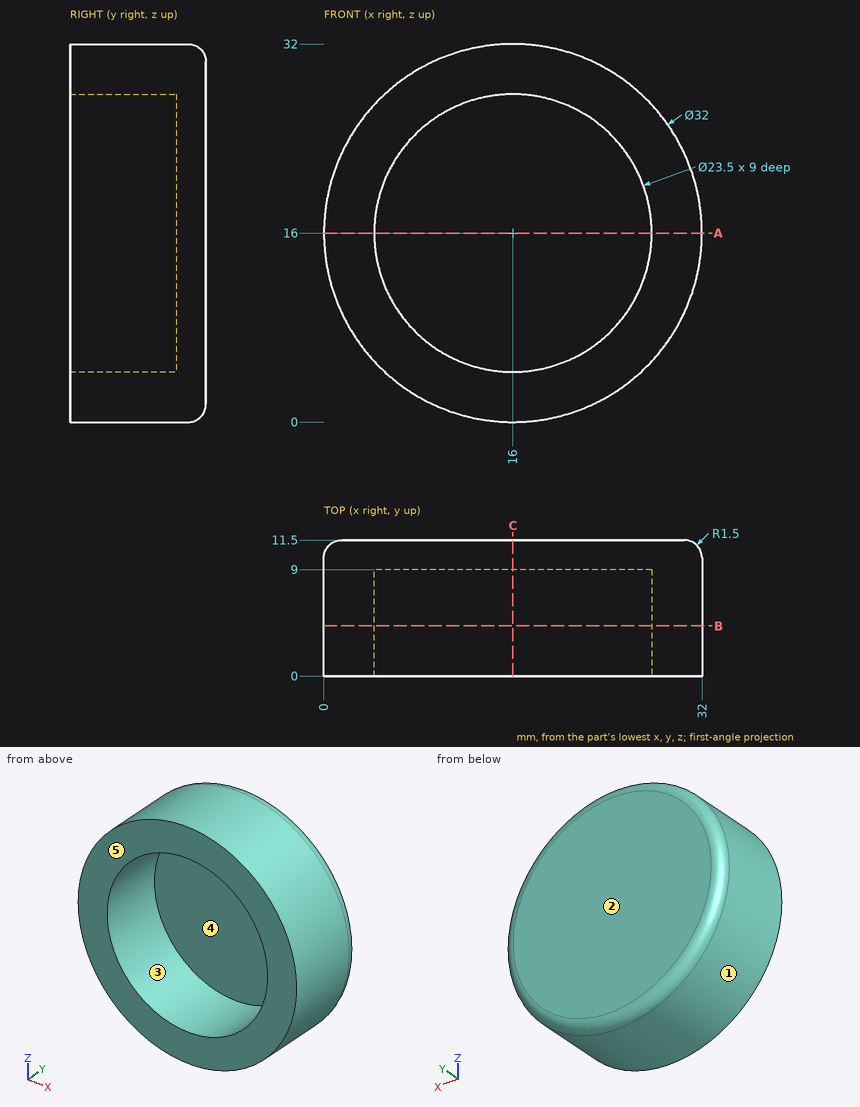
Check sheet for the drawn part. Datum: minimum x, y, z corner. Units: mm. A direction names the side the tool comes from. Give positions to 0.01 mm unless a question says otherwise; leave off trailing zeros. Loops run counter-clockwise (first coordinate to the right, second up) from the corner with the lowest first, then second, coordinate; pieces in that order, holes last.
1) Depth check by flat-ended pin: pin 1 Ø6 at (y, z) = (9, 25) entering from -X; pin 2 Ø1 at (x, y) = (18, 3) entering from -Z; pin 3 Ø6 at (x, y) = (4.5, 4) entering from -Z. Enter the tip coordinate at first touch or a pass-through.
2) Sectioned sample at B-B, the plane y = 4.25. Enter the section's corners in (x, z).
3) Set-up check for the marked faces 4 and 5: record each of +Z, -Z, +X, -X, +Y, -Y from which the full face is reachable in a straight line by a thin tool's end or side.
4) Thickness scan on line 1 along Z through (x, y) = (16, 2); line 2 along Z through (x, y) = (8, 8); line 3 along X through (y, z) = (7.5, 21). Record the ranges inside material, lowest first.
5) Draft check along Z on the marked faces 1, 2 and 3. Enter one of: pulls with the +Z half, pulls with the -Z half, needs draft (parallel to the pull), parting line crosses it, or undercut.
6) Sectioned sample at C-C, the plane x = 16. Enter the section's corners in (y, z).
7) Sectioned sample at A-A, the plane z = 16. Enter the section's corners in (x, y).
Answers:
1. pin 1: stops at x = 1.17
1. pin 2: stops at z = 0.07
1. pin 3: stops at z = 2.44
2. outline: circle Ø32 at (16, 16); hole circle Ø23.5 at (16, 16)
3. face 4: -Y
3. face 5: +Z, -Z, +X, -X, -Y
4. line 1: z = 0 to 4.25, 27.75 to 32
4. line 2: z = 2.14 to 7.39, 24.61 to 29.86
4. line 3: x = 0.8 to 5.37, 26.63 to 31.2
5. face 1: parting line crosses it
5. face 2: needs draft
5. face 3: undercut
6. outline: (0, 0) - (10, 0) arc R1.5 ccw to (11.5, 1.5) - (11.5, 30.5) arc R1.5 ccw to (10, 32) - (0, 32) - (0, 27.75) - (9, 27.75) - (9, 4.25) - (0, 4.25) - close
7. outline: (0, 0) - (4.25, 0) - (4.25, 9) - (27.75, 9) - (27.75, 0) - (32, 0) - (32, 10) arc R1.5 ccw to (30.5, 11.5) - (1.5, 11.5) arc R1.5 ccw to (0, 10) - close
